Geometry check sheet. Reference: the model listing, model coordinates, mm. Face numbers are marked on the shaded views. A direction names the side the tool comes from. Round coordinates to 2 decimals unless told otherwise and drop trailing zeros. Write each loop counter-clockwise with the first axis right and the second up, starting at its lowest first coordinate (ties: lowest second). Pieces come first, ordered by that corner, then holes. Notation, with made-up numbers: M -6.5,-27.75 L 31.5,-27.75 A16 cw 31.5,0.25 Z; hole C 68.25,-10 d10. An arc over 180 degrees is marked long. One line per item, written item: value. Start each with the question number.
1. Section check A-A (x = 0). Record the boundary of the cut face in (y, z), and give its area (3 significant figures).
2. Depth check by flat-ended pin: P1, Ø2, axis at x = 29, z = 12.5, coming from the -Y side; P2, Ø10, axis at y = -41.5, z = 8, coming from the -X side; P3, Ø6.5, axis at y = -62, z = 21, coming from the -X side; P4, Ø8, axis at x = 0, y = -21, coming from the +Z side. Enter the tip coordinate at first touch or a pass-through.
3. Access from +Z, -Z, +X, -X, +Y, -Y to the whole of each face (thin tool, end or side, straight path). Record for the marked faces 1, 2, 3 and 4.
4. Scan lines: probe 1 along X at (y, z) = (0, 3); probe 2 along Y at (x, z) = (0, 8.5). Record each from-to range of solid material in increasing order. Write a range as [from, to].
5. Release check for a two-part mould opening along Y. For the marked faces 5, 6 and 7 record: pulls with the +Y half, pulls with the -Y half, needs draft (parallel to the pull), parting line crosses it, or undercut.
6. Section check C-C (z = 9). Record the boundary of the cut face in (x, y), and give its area (3 significant figures).
7. Section check B-B (y = 0). Record the boundary of the cut face in (x, z).
8. Section check D-D (z = 17). Record the boundary of the cut face in (x, y), and give its area (3 significant figures).
from build123d import *

# Parameters (mm, degrees)
F0_R     = 55
F1_DEPTH = 14
F2_R     = 52
F3_DEPTH = 7
F4_R     = 6
F5_DEPTH = 14.001
F7_DEPTH = 20


with BuildPart() as f1:
    # F0 (on Top) → F1 (new body)
    with BuildSketch(Plane.XY):
        Circle(F0_R)
    extrude(amount=F1_DEPTH)

    # F2 (on face) → F3 (cut)
    with BuildSketch(Plane(origin=(0, 0, 0), x_dir=(1, 0, 0), z_dir=(0, 0, -1))):
        Circle(F2_R)
    extrude(amount=-F3_DEPTH, mode=Mode.SUBTRACT)

    # F4 (on face) → F5 (cut, through all)
    with BuildSketch(Plane.XY.offset(14)):
        with Locations((0, -25)):
            Circle(F4_R)
    extrude(amount=-F5_DEPTH, mode=Mode.SUBTRACT)

    # F6 (on face) → F7 (join)
    with BuildSketch(Plane.XY.offset(14)):
        with BuildLine():
            Line((-15, -65), (-15, -52.915026))
            ThreePointArc((-15, -52.915026), (-16.50511, -52.465049), (-17.996755, -51.97227))
            ThreePointArc((-17.996755, -51.97227), (-17.999189, -52.128262), (-18, -52.284271))
            Line((-18, -52.284271), (-18, -65))
            Line((-18, -65), (-15, -65))
        make_face()
        with BuildLine():
            Line((-6, -35), (-6, -25))
            ThreePointArc((-6, -25), (0, -19), (6, -25))
            Line((6, -25), (6, -35))
            ThreePointArc((6, -35), (6.608964, -38.061467), (8.343146, -40.656854))
            Line((8.343146, -40.656854), (11.485281, -43.79899))
            ThreePointArc((11.485281, -43.79899), (14.086554, -47.69207), (15, -52.284271))
            Line((15, -52.284271), (15, -52.915026))
            ThreePointArc((15, -52.915026), (16.50511, -52.465049), (17.996755, -51.97227))
            ThreePointArc((17.996755, -51.97227), (16.797741, -46.400197), (13.606602, -41.67767))
            Line((13.606602, -41.67767), (10.464466, -38.535534))
            ThreePointArc((10.464466, -38.535534), (9.380602, -36.913417), (9, -35))
            Line((9, -35), (9, -25))
            ThreePointArc((9, -25), (0, -16), (-9, -25))
            Line((-9, -25), (-9, -35))
            ThreePointArc((-9, -35), (-9.380602, -36.913417), (-10.464466, -38.535534))
            Line((-10.464466, -38.535534), (-13.606602, -41.67767))
            ThreePointArc((-13.606602, -41.67767), (-16.797741, -46.400197), (-17.996755, -51.97227))
            ThreePointArc((-17.996755, -51.97227), (-16.50511, -52.465049), (-15, -52.915026))
            Line((-15, -52.915026), (-15, -52.284271))
            ThreePointArc((-15, -52.284271), (-14.086554, -47.69207), (-11.485281, -43.79899))
            Line((-11.485281, -43.79899), (-8.343146, -40.656854))
            ThreePointArc((-8.343146, -40.656854), (-6.608964, -38.061467), (-6, -35))
        make_face()
        with BuildLine():
            ThreePointArc((17.996755, -51.97227), (16.50511, -52.465049), (15, -52.915026))
            Line((15, -52.915026), (15, -65))
            Line((15, -65), (18, -65))
            Line((18, -65), (18, -52.284271))
            ThreePointArc((18, -52.284271), (17.999189, -52.128262), (17.996755, -51.97227))
        make_face()
    extrude(amount=F7_DEPTH)


solid = f1.part
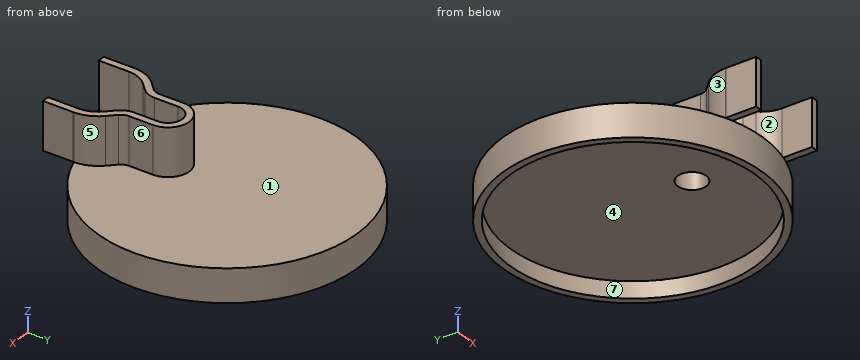
Result sheet:
1. outline: M -55,0 L -52,0 L -52,7 L -31,7 L -31,14 L -55,14 Z; M -19,7 L 52,7 L 52,0 L 55,0 L 55,14 L -16,14 L -16,34 L -19,34 Z
1. area: 788 mm2
2. P1: stops at y = -47.34
2. P2: stops at x = -41.14
2. P3: stops at x = -18
2. P4: stops at z = 34
3. face 1: +Z, +Y
3. face 2: +Z, -Y
3. face 3: +Z, -X, +Y
3. face 4: -Z
4. probe 1: x = [-55, -52], [52, 55]
4. probe 2: y = [-55, -31], [-19, 55]
5. face 5: pulls with the +Y half
5. face 6: needs draft
5. face 7: undercut
6. outline: C 0,0 d110; hole C 0,-25 d12
6. area: 9,390 mm2
7. outline: M -55,0 L -52,0 L -52,7 L 52,7 L 52,0 L 55,0 L 55,14 L -55,14 Z
8. outline: M -18,-65 L -15,-65 L -15,-52.28 A12 cw -11.49,-43.8 L -8.34,-40.66 A8 ccw -6,-35 L -6,-25 A6 cw 6,-25 L 6,-35 A8 ccw 8.34,-40.66 L 11.49,-43.8 A12 cw 15,-52.28 L 15,-65 L 18,-65 L 18,-52.28 A15 ccw 18,-51.97 A15 ccw 13.61,-41.68 L 10.46,-38.54 A5 cw 9,-35 L 9,-25 A9 ccw -9,-25 L -9,-35 A5 cw -10.46,-38.54 L -13.61,-41.68 A15 ccw -18,-51.97 A15 ccw -18,-52.28 Z
8. area: 328 mm2
